Design review of the part shown in the three views and the two pictorial views. Dimensions are in mm from the part's minimum x, y and z. Give positions to 0.01 mm unless a question says otherwise; leave off trailing zeros. Loops run counter-clockwise (first coordinate to the right, second up) from the corner with the lowest first, then second, coordinate; pieces in that order, holes last. Notation, with made-up numbers: (-4.75, 2.25) - (53.25, 2.25) arc R14 ccw to (53.25, 19.25) - close; hole circle Ø8 at (71.25, 80). An arc over 180 degrees is marked (long way). Put each result on its own line as item: value. Start each with the question number.
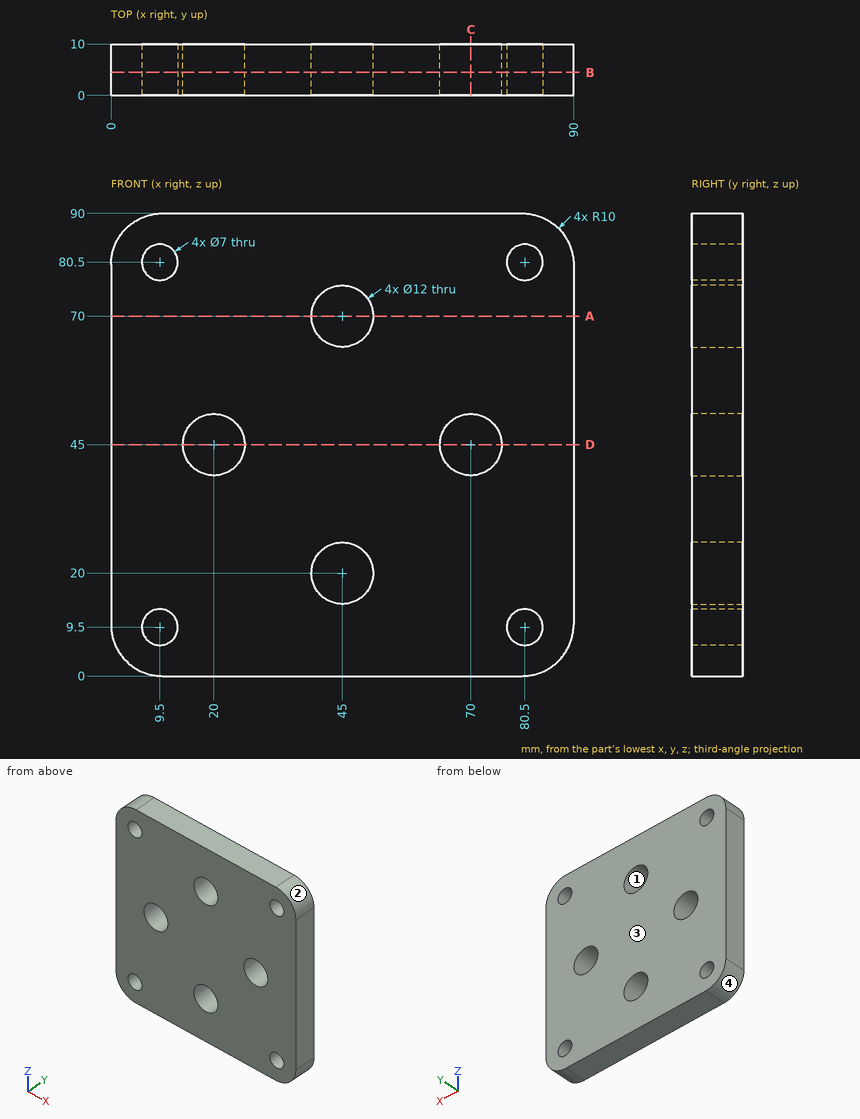
1) Take a section at A-A on z = 70. State the section outline as (x, y) points.
2) Mouldability with a two-part tool opening along X and no side actions: class the marked faces 1, 2, 3 and 4 as released by +X, released by -X, zero draft, split by the parting line, or undercut.
3) Take a section at D-D on z = 45. State the section outline as (x, y) points, and give its area (3 significant figures).
4) Wall thickness on probe 1 along X at (y, z) = (6, 80.5); probe 2 along X at (y, z) = (4.5, 45); probe 3 along X at (y, z) = (7.75, 20): over which ranges is each line inside the solid? List them lowest first.
5) Take a section at C-C on x = 70. State the section outline as (y, z) points.
6) Take a section at B-B on y = 4.5. State how many separate pieces and enclosed holes the cut face has, and give its area (3 significant figures).
7) Insertion check: P1, Ø7, axis at x = 45, z = 20, coming from the +Y side. The pin has a flat end and moves straight along its axis. Give the tip position at first contact, or say it passes through.
Answers follow:
1. outline: (0, 0) - (39, 0) - (39, 10) - (0, 10) - close; (51, 0) - (90, 0) - (90, 10) - (51, 10) - close
2. face 1: undercut
2. face 2: released by +X
2. face 3: zero draft
2. face 4: released by -X
3. outline: (0, 0) - (14, 0) - (14, 10) - (0, 10) - close; (26, 0) - (64, 0) - (64, 10) - (26, 10) - close; (76, 0) - (90, 0) - (90, 10) - (76, 10) - close
3. area: 660 mm2
4. probe 1: 0.01 to 6, 13 to 77, 84 to 89.99
4. probe 2: 0 to 14, 26 to 64, 76 to 90
4. probe 3: 0 to 39, 51 to 90
5. outline: (0, 0) - (10, 0) - (10, 39) - (0, 39) - close; (0, 51) - (10, 51) - (10, 90) - (0, 90) - close
6. separate pieces: 1
6. enclosed holes: 8
6. area: 7,410 mm2
7. P1: through
